Geometry check sheet. Reference: the model listing, model coordinates, mm. Face numbers are marked on the shaded views. A direction names the side the tool comes from. Give positions to 0.01 mm unless a question says otherwise; leave off trailing zeros. Write each loop counter-clockwise with the first axis right and the second up, starting at its lowest first coordinate (ties: lowest second). Pieces come first, ordered by that corner, then holes.
(1) Mould release check, pull along Z, two halves, no side actions. Record for the marked faces 1, 2 and 3: +Z half, -Z half, draft (parallel to the pull), parting line (faces both ways), or undercut.
(2) Thickness scan on line 1 along X through (y, z) = (166, 0); line 2 along Y through (x, z) = (-120, 75); line 3 along X through (y, z) = (56, 100). Record the ranges inside material, lowest first.
(3) Tool access check on the marked faces 4, 5, 6, 7 and 8. Record the directions out of +Z, -Z, +X, -X, +Y, -Y that give a thin tool (end or side, any length) a straight path to the whole face; none if there is none.
(4) Depth check by flat-ended pin: P1, Ø8, axis at y = 142, z = -186.5, coming from the +X side; P2, Ø1.5, axis at x = -85.5, z = -33, coming from the +Y side; P3, Ø1, axis at y = 110, z = -189.5, coming from the +X side. Enter the tip coordinate at first touch or a pass-through.
(5) Cross-section at B-B (y = 170). Record the boundary of the cut face in (x, z).
(6) Cross-section at A-A (y = 77.5). Count the separate pieces of the cut face and the enclosed holes in it, and give its area (3 significant figures).
```python
from build123d import *

# Parameters (mm, degrees)
SKETCH1_R           = 276
SKETCH1_R_2         = 16.5
BOSS_EXTRUDE1_DEPTH = 12
SKETCH2_R           = 36.5
SKETCH2_R_2         = 16.5
BOSS_EXTRUDE2_DEPTH = 104
SKETCH4_R           = 276
SKETCH4_R_2         = 96
BOSS_EXTRUDE6_DEPTH = 12
BOSS_EXTRUDE7_DEPTH = 24
SKETCH6_R           = 114
SKETCH6_R_2         = 96
BOSS_EXTRUDE8_DEPTH = 72
FILLET1_R           = 14
SKETCH7_R           = 36.5
SKETCH7_R_2         = 16.5
BOSS_EXTRUDE9_DEPTH = 84


with BuildPart() as part:
    # Sketch1 → Boss-Extrude1 (new body)
    with BuildSketch(Plane(origin=(0, 0, 0), x_dir=(1, 0, 0), z_dir=(0, 1, 0))):
        with Locations(Location((0, 0, 0), (0, 0, 270))):
            Circle(SKETCH1_R)
        with Locations(Location((0, 0, 0), (0, 0, 270))):
            Circle(SKETCH1_R_2, mode=Mode.SUBTRACT)
    extrude(amount=BOSS_EXTRUDE1_DEPTH)

    # Sketch2 → Boss-Extrude2 (add)
    # profile 1 of 9: a face of its own
    with BuildSketch(Plane(origin=(0, 12, 0), x_dir=(1, 0, 0), z_dir=(0, 1, 0))):
        with Locations(Location((0, 0, 0), (0, 0, 90))):
            Circle(SKETCH2_R)
        with Locations(Location((0, 0, 0), (0, 0, 270))):
            Circle(SKETCH2_R_2, mode=Mode.SUBTRACT)
    # profile 2 of 9: a face of its own
    with BuildSketch(Plane(origin=(0, 12, 0), x_dir=(1, 0, 0), z_dir=(0, 1, 0))):
        with BuildLine():
            ThreePointArc((15.99428821, -144.42748644), (0.354884611, -128.003936206), (-15.997509824, -143.717724529))
            ThreePointArc((-15.997509824, -143.717724529), (-46.818792615, -205.414811389), (-114.180459904, -220.209667925))
            ThreePointArc((-114.180459904, -220.209667925), (-123.660150756, -225.693034374), (-118.785216252, -235.499504679))
            ThreePointArc((-118.785216252, -235.499504679), (-27.982252168, -224.613228291), (15.99428821, -144.42748644))
        make_face()
    # profile 3 of 9: a face of its own
    with BuildSketch(Plane(origin=(0, 12, 0), x_dir=(1, 0, 0), z_dir=(0, 1, 0))):
        with BuildLine():
            ThreePointArc((-90.815985398, -113.435324705), (-90.261509995, -90.763392625), (-112.93572527, -90.311829913))
            ThreePointArc((-112.93572527, -90.311829913), (-178.356091834, -112.144320345), (-236.44952695, -74.973971996))
            ThreePointArc((-236.44952695, -74.973971996), (-247.030006234, -72.14814391), (-250.517128641, -82.529464808))
            ThreePointArc((-250.517128641, -82.529464808), (-178.61197713, -139.039096608), (-90.815985398, -113.435324705))
        make_face()
    # profile 4 of 9: a face of its own
    with BuildSketch(Plane(origin=(0, 12, 0), x_dir=(1, 0, 0), z_dir=(0, 1, 0))):
        with BuildLine():
            ThreePointArc((-144.42748644, -15.99428821), (-128.003936206, -0.354884611), (-143.717724529, 15.997509824))
            ThreePointArc((-143.717724529, 15.997509824), (-205.414811389, 46.818792615), (-220.209667925, 114.180459904))
            ThreePointArc((-220.209667925, 114.180459904), (-225.693034374, 123.660150756), (-235.499504679, 118.785216252))
            ThreePointArc((-235.499504679, 118.785216252), (-224.613228291, 27.982252168), (-144.42748644, -15.99428821))
        make_face()
    # profile 5 of 9: a face of its own
    with BuildSketch(Plane(origin=(0, 12, 0), x_dir=(1, 0, 0), z_dir=(0, 1, 0))):
        with BuildLine():
            ThreePointArc((-113.435324705, 90.815985398), (-90.763392625, 90.261509995), (-90.311829913, 112.93572527))
            ThreePointArc((-90.311829913, 112.93572527), (-112.144320345, 178.356091834), (-74.973971996, 236.44952695))
            ThreePointArc((-74.973971996, 236.44952695), (-72.14814391, 247.030006234), (-82.529464808, 250.517128641))
            ThreePointArc((-82.529464808, 250.517128641), (-139.039096608, 178.61197713), (-113.435324705, 90.815985398))
        make_face()
    # profile 6 of 9: a face of its own
    with BuildSketch(Plane(origin=(0, 12, 0), x_dir=(1, 0, 0), z_dir=(0, 1, 0))):
        with BuildLine():
            ThreePointArc((-15.99428821, 144.42748644), (-0.354884611, 128.003936206), (15.997509824, 143.717724529))
            ThreePointArc((15.997509824, 143.717724529), (46.818792615, 205.414811389), (114.180459904, 220.209667925))
            ThreePointArc((114.180459904, 220.209667925), (123.660150756, 225.693034374), (118.785216252, 235.499504679))
            ThreePointArc((118.785216252, 235.499504679), (27.982252168, 224.613228291), (-15.99428821, 144.42748644))
        make_face()
    # profile 7 of 9: a face of its own
    with BuildSketch(Plane(origin=(0, 12, 0), x_dir=(1, 0, 0), z_dir=(0, 1, 0))):
        with BuildLine():
            ThreePointArc((90.815985398, 113.435324705), (90.261509995, 90.763392625), (112.93572527, 90.311829913))
            ThreePointArc((112.93572527, 90.311829913), (178.356091834, 112.144320345), (236.44952695, 74.973971996))
            ThreePointArc((236.44952695, 74.973971996), (247.030006234, 72.14814391), (250.517128641, 82.529464808))
            ThreePointArc((250.517128641, 82.529464808), (178.61197713, 139.039096608), (90.815985398, 113.435324705))
        make_face()
    # profile 8 of 9: a face of its own
    with BuildSketch(Plane(origin=(0, 12, 0), x_dir=(1, 0, 0), z_dir=(0, 1, 0))):
        with BuildLine():
            ThreePointArc((144.42748644, 15.99428821), (128.003936206, 0.354884611), (143.717724529, -15.997509824))
            ThreePointArc((143.717724529, -15.997509824), (205.414811389, -46.818792615), (220.209667925, -114.180459904))
            ThreePointArc((220.209667925, -114.180459904), (225.693034374, -123.660150756), (235.499504679, -118.785216252))
            ThreePointArc((235.499504679, -118.785216252), (224.613228291, -27.982252168), (144.42748644, 15.99428821))
        make_face()
    # profile 9 of 9: a face of its own
    with BuildSketch(Plane(origin=(0, 12, 0), x_dir=(1, 0, 0), z_dir=(0, 1, 0))):
        with BuildLine():
            ThreePointArc((113.435324705, -90.815985398), (90.763392625, -90.261509995), (90.311829913, -112.93572527))
            ThreePointArc((90.311829913, -112.93572527), (112.144320345, -178.356091834), (74.973971996, -236.44952695))
            ThreePointArc((74.973971996, -236.44952695), (72.14814391, -247.030006234), (82.529464808, -250.517128641))
            ThreePointArc((82.529464808, -250.517128641), (139.039096608, -178.61197713), (113.435324705, -90.815985398))
        make_face()
    extrude(amount=BOSS_EXTRUDE2_DEPTH)

    # Sketch4 → Boss-Extrude6 (add)
    with BuildSketch(Plane(origin=(0, 116, 0), x_dir=(1, 0, 0), z_dir=(0, 1, 0))):
        with Locations(Location((0, 0, 0), (0, 0, 270))):
            Circle(SKETCH4_R)
        with Locations(Location((0, 0, 0), (0, 0, 270))):
            Circle(SKETCH4_R_2, mode=Mode.SUBTRACT)
    extrude(amount=BOSS_EXTRUDE6_DEPTH)

    # Sketch5 → Boss-Extrude7 (add)
    with BuildSketch(Plane(origin=(0, 128, 0), x_dir=(1, 0, 0), z_dir=(0, 1, 0))):
        with BuildLine():
            ThreePointArc((170.830485383, -212.939679185), (163.2534903, -137.16642294), (106.076926652, -86.868930102))
            ThreePointArc((106.076926652, -86.868930102), (80.332659261, -99.281912309), (93.285108283, -124.759029396))
            ThreePointArc((93.285108283, -124.759029396), (135.370747242, -156.776062336), (147.364000345, -208.278035938))
            ThreePointArc((147.364000345, -208.278035938), (156.943786511, -221.449251949), (170.830485383, -212.939679185))
        make_face()
        with BuildLine():
            ThreePointArc((-212.939679185, -170.830485383), (-137.16642294, -163.2534903), (-86.868930102, -106.076926652))
            ThreePointArc((-86.868930102, -106.076926652), (-99.281912309, -80.332659261), (-124.759029396, -93.285108283))
            ThreePointArc((-124.759029396, -93.285108283), (-156.776062336, -135.370747242), (-208.278035938, -147.364000345))
            ThreePointArc((-208.278035938, -147.364000345), (-221.449251949, -156.943786511), (-212.939679185, -170.830485383))
        make_face()
        with BuildLine():
            ThreePointArc((-170.830485383, 212.939679185), (-163.2534903, 137.16642294), (-106.076926652, 86.868930102))
            ThreePointArc((-106.076926652, 86.868930102), (-80.332659261, 99.281912309), (-93.285108283, 124.759029396))
            ThreePointArc((-93.285108283, 124.759029396), (-135.370747242, 156.776062336), (-147.364000345, 208.278035938))
            ThreePointArc((-147.364000345, 208.278035938), (-156.943786511, 221.449251949), (-170.830485383, 212.939679185))
        make_face()
        with BuildLine():
            ThreePointArc((212.939679185, 170.830485383), (137.16642294, 163.2534903), (86.868930102, 106.076926652))
            ThreePointArc((86.868930102, 106.076926652), (99.281912309, 80.332659261), (124.759029396, 93.285108283))
            ThreePointArc((124.759029396, 93.285108283), (156.776062336, 135.370747242), (208.278035938, 147.364000345))
            ThreePointArc((208.278035938, 147.364000345), (221.449251949, 156.943786511), (212.939679185, 170.830485383))
        make_face()
    extrude(amount=BOSS_EXTRUDE7_DEPTH)

    # Sketch6 → Boss-Extrude8 (add)
    with BuildSketch(Plane(origin=(0, 128, 0), x_dir=(1, 0, 0), z_dir=(0, 1, 0))):
        with Locations(Location((0, 0, 0), (0, 0, 270))):
            Circle(SKETCH6_R)
        with Locations(Location((0, 0, 0), (0, 0, 270))):
            Circle(SKETCH6_R_2, mode=Mode.SUBTRACT)
    extrude(amount=BOSS_EXTRUDE8_DEPTH)

    # Fillet1
    fillet1_edges = [part.edges().sort_by_distance(p)[0] for p in [
        (0, 12, 36.5),
    ]]
    fillet(fillet1_edges, radius=FILLET1_R)

    # Sketch7 → Boss-Extrude9 (add)
    with BuildSketch(Plane(origin=(0, 116, 0), x_dir=(1, 0, 0), z_dir=(0, 1, 0))):
        with Locations(Location((0, 0, 0), (0, 0, 90))):
            Circle(SKETCH7_R)
        with Locations(Location((0, 0, 0), (0, 0, 270))):
            Circle(SKETCH7_R_2, mode=Mode.SUBTRACT)
    extrude(amount=BOSS_EXTRUDE9_DEPTH)


solid = part.part
```
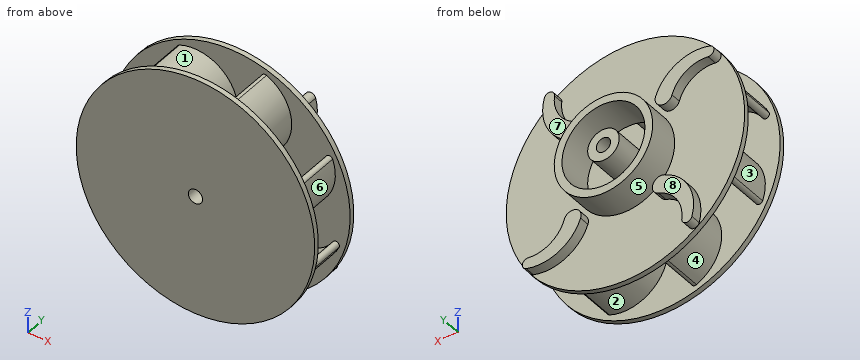
Reply:
1. face 1: +Z half
1. face 2: -Z half
1. face 3: undercut
2. line 1: x = -114 to -96, -36.5 to -16.5, 16.5 to 36.5, 96 to 114
2. line 2: y = 0 to 12, 116 to 128
2. line 3: x = -240.25 to -211.83, -125.16 to -85.93, 85.93 to 121.15, 222.21 to 240.46
3. face 4: none
3. face 5: +Y
3. face 6: +X
3. face 7: +Z, +X, +Y
3. face 8: -Z, -X, +Y
4. P1: stops at x = -146.1
4. P2: stops at y = 12
4. P3: stops at x = 31.76
5. outline: circle Ø228 at (0, 0); circle Ø73 at (0, 0); hole circle Ø192 at (0, 0); hole circle Ø33 at (0, 0)
6. separate pieces: 9
6. enclosed holes: 1
6. area: 41,500 mm2
